For this review, use the dimensioned drawing (mm, ordinates from the lowest corner) and the shaded views. A direction names the side the tool comes from. Coordinates: 2 decimals unless noted, no trailing zeros. Order: outer loops, then holes, each group sorted by start corner. A loop starts at its lowest first (then second) coordinate and runs counter-clockwise, first axis right, second up. Notation, with made-up numbers: (4.5, 48) -> (52.5, 48) arc R22 ccw to (52.5, 80) -> close; hole circle Ø2 at (29.25, 66.25). An arc over 180 degrees is marked (long way). Return JSON: item names as keys, results as strings. Group by question number.
Item 1: Take a section at A-A (x = 8.5). Write out the cut boundary in (y, z).
Item 2: Take a section at C-C (y = 8.5). Write out the cut boundary in (x, z).
Item 3: Take a section at D-D (x = 20.5). Write out the cut boundary in (y, z).
Item 4: Machinability: for the marked faces 1, 2 and 3, which of the approach directions +Z, -Z, +X, -X, +Y, -Y give a long, thin tool a straight path to every point of the face, cutting with its end or side? Answer none if there is none.
Item 5: For line 1 along X through (y, z) = (17.5, 3.5); line 2 along Y through (x, z) = (5.5, 3.5); line 3 along Z through (x, y) = (3.75, 5), list the stretches that pass through material, from the lowest coordinate up.
Item 6: Take a section at B-B (z = 21). Write out the cut boundary in (x, y), then the cut area to 3 significant figures.
Item 7: Insertion check: pin 1 (6 mm diameter, centred on x = 9, y = 24, fed in from -Z); pin 2 (1 mm diameter, centred on x = 22.5, y = 11.5, fed in from +Z); pin 3 (12.5 mm diameter, centred on x = 9, z = 20.5, fed in from -Y). Each pin has a flat end and moves straight along its axis. Give the tip position at first contact, or say it passes through.
Item 8: Draft analysis for pull direction Y (two halves, no side actions). For the marked faces 4, 5, 6 and 7, state which applies: +Y half, -Y half, draft (parallel to the pull), parting line (faces both ways), or undercut.
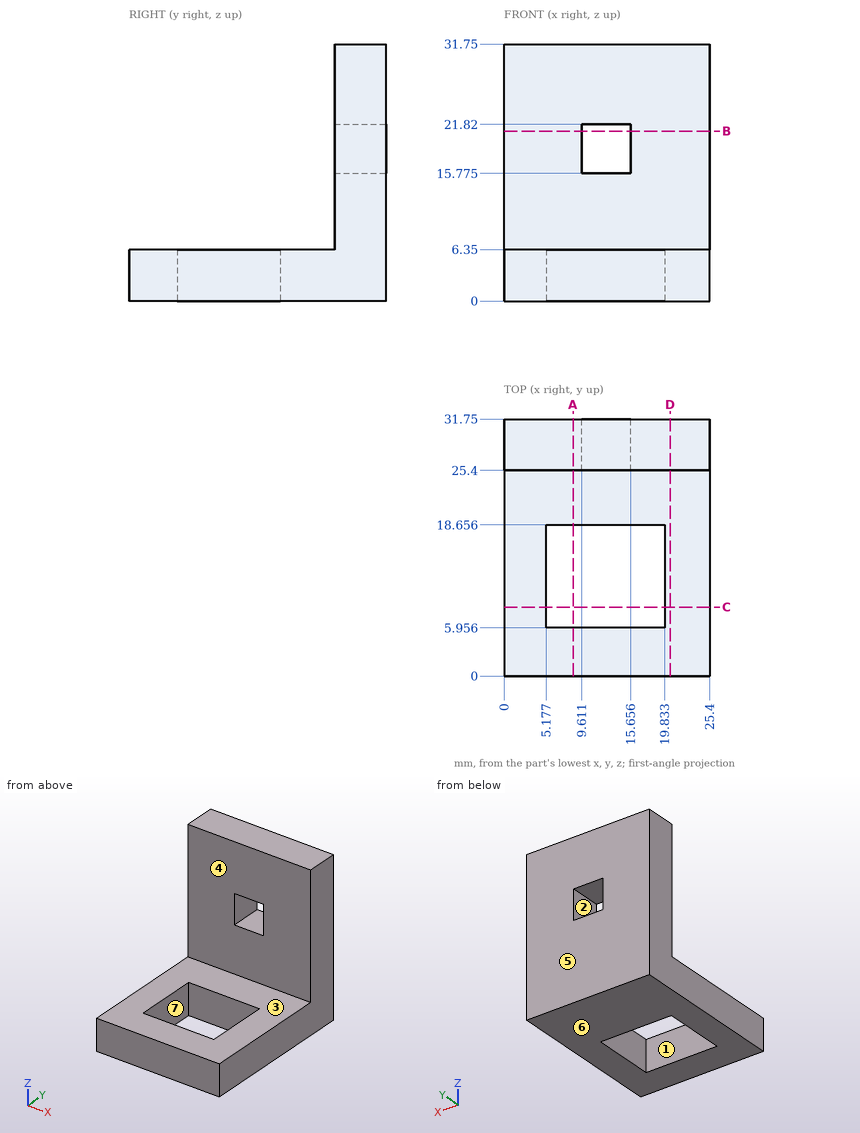
Findings below:
{
 "1": {"outline": "(0, 0) -> (5.96, 0) -> (5.96, 6.35) -> (0, 6.35) -> close; (18.66, 0) -> (31.75, 0) -> (31.75, 31.75) -> (25.4, 31.75) -> (25.4, 6.35) -> (18.66, 6.35) -> close"},
 "2": {"outline": "(0, 0) -> (5.18, 0) -> (5.18, 6.35) -> (0, 6.35) -> close; (19.83, 0) -> (25.4, 0) -> (25.4, 6.35) -> (19.83, 6.35) -> close"},
 "3": {"outline": "(0, 0) -> (31.75, 0) -> (31.75, 31.75) -> (25.4, 31.75) -> (25.4, 6.35) -> (0, 6.35) -> close"},
 "4": {"face 1": "+Z, -Z", "face 2": "+Y, -Y", "face 3": "+Z, +X, -X, -Y"},
 "5": {"line 1": "x = 0 to 5.18, 19.83 to 25.4", "line 2": "y = 0 to 5.96, 18.66 to 31.75", "line 3": "z = 0 to 6.35"},
 "6": {"outline": "(0, 25.4) -> (9.61, 25.4) -> (9.61, 31.75) -> (0, 31.75) -> close; (15.66, 25.4) -> (25.4, 25.4) -> (25.4, 31.75) -> (15.66, 31.75) -> close", "area": "123 mm2"},
 "7": {"pin 1": "stops at z = 0", "pin 2": "stops at z = 6.35", "pin 3": "stops at y = 25.4"},
 "8": {"face 4": "-Y half", "face 5": "+Y half", "face 6": "draft", "face 7": "undercut"}
}
